from build123d import *

# Parameters (mm, degrees)
BOSS_EXTRUDE5_DEPTH = 4
SKETCH8_W           = 31.9
SKETCH8_H           = 15.8
BOSS_EXTRUDE8_DEPTH = 4.7


with BuildPart() as part:
    # Sketch1 → Boss-Extrude5 (new body)
    with BuildSketch(Plane(origin=(0, 0, 0), x_dir=(1, 0, 0), z_dir=(0, 1, 0))):
        Polygon((-17.521212205, 5.796054243), (-17.521212205, -6.003945757), (-17.521212205, -8.003945757), (14.378787795, -8.003945757), (14.378787795, -6.003945757), (14.378787795, 5.796054243), (14.378787795, 7.796054243), (-17.521212205, 7.796054243), align=None)
        with BuildLine():
            Line((-0.998289948, -2.601375998), (-1.554401677, -2.601375998))
            ThreePointArc((-1.554401677, -2.601375998), (-12.793150429, -0.101375998), (-1.554401677, 2.398624002))
            Line((-1.554401677, 2.398624002), (-0.998289948, 2.398624002))
            ThreePointArc((-0.998289948, 2.398624002), (1.501710052, -0.101375998), (-0.998289948, -2.601375998))
        make_face(mode=Mode.SUBTRACT)
    extrude(amount=BOSS_EXTRUDE5_DEPTH)

    # Sketch8 → Boss-Extrude8 (add)
    with BuildSketch(Plane(origin=(0, 4, 0), x_dir=(1, 0, 0), z_dir=(0, 1, 0))):
        with Locations((-1.571212205, -0.103945757)):
            Rectangle(SKETCH8_W, SKETCH8_H)
        Polygon((-6.895720189, 5.796054243), (-12.793150429, 5.796054243), (-12.793150429, -0.101375998), (-12.793150429, -5.998806238), (-6.895720189, -5.998806238), (9.704279811, -5.998806238), (9.704279811, 5.796054243), align=None, mode=Mode.SUBTRACT)
    extrude(amount=BOSS_EXTRUDE8_DEPTH)


solid = part.part
Design review of the part built by this model. Coordinates are the model's own, in mm. A direction names the side the tool comes from. Round coordinates to 2 decimals unless told otherwise and drop trailing zeros. Order: outer loops, then holes, each group sorted by start corner. A loop starts at its lowest first (then second) coordinate and runs counter-clockwise, first axis right, second up. Notation, with made-up numbers: M -12.5,18 L 0.5,18 A22 cw 0.5,47 Z; hole C 57.25,55.25 d4. An arc over 180 degrees is marked long. Answer as CSV lines item,"result". Start each with the question number.
1) The part is to be moulded in two halves that separate along Z. For faces 1 (the face through (9.704, 6, 0)), 2 (the face through (14.379, 4, 0)), 3 (the face through (-2, 4, 8.004)), 4 (the face through (-12.793, 6, 0)), say which applies: +Z half, -Z half, draft (parallel to the pull), parting line (faces both ways), or undercut.
2) For pin 1 Ø1.8 at (x, z) = (-10, 3) entering from +Y; pin 2 Ø6 at (x, z) = (3.5, 1) entering from +Y, all flat-tipped, find the tip position at first contact; note any pin that passes through.
3) Add section D-D (x = 8). Give the boundary of the cut face in (y, z), then the cut area to 3 significant figures.
4) Tool access review of faces 5 (the face through (1.5, 2, 0)), 6 (the face through (-2, 4, -7.796)), 7 (the face through (-2, 6, -5.796)): name each direction out of +Z, -Z, +X, -X, +Y, -Y from which nothing blocks a thin tool from reaching the whole face with its end or side.
5) Wall thickness on line 1 along Z through (x, y) = (3, 8.5); line 2 along X through (y, z) = (6.75, 3.75); line 3 along Y through (x, z) = (4, -5.25): over which ranges is each line inside the solid? List them lowest first. Write a range as [from, to].
6) Add section B-B (x = -0.5). Give the boundary of the cut face in (y, z).
7) Add section A-A (y = 6.5). Give the boundary of the cut face in (x, z), then the cut area to 3 significant figures.
Resolved:
1,face 1,"undercut"
1,face 2,"draft"
1,face 3,"+Z half"
1,face 4,"undercut"
2,pin 1,"through"
2,pin 2,"y = 4"
3,outline,"M 0,-7.8 L 8.7,-7.8 L 8.7,-5.8 L 4,-5.8 L 4,6 L 8.7,6 L 8.7,8 L 0,8 Z"
3,area,"82.0 mm^2"
4,face 5,"+Y, -Y"
4,face 6,"-Z, +X, -X, +Y, -Y"
4,face 7,"+Y"
5,line 1,"[-7.8, -5.8], [6, 8]"
5,line 2,"[-17.52, -12.79], [9.7, 14.38]"
5,line 3,"[0, 4]"
6,outline,"M 0,-7.8 L 8.7,-7.8 L 8.7,-5.8 L 4,-5.8 L 4,-2.35 L 0,-2.35 Z; M 0,2.55 L 4,2.55 L 4,6 L 8.7,6 L 8.7,8 L 0,8 Z"
7,outline,"M -17.52,-7.8 L 14.38,-7.8 L 14.38,8 L -17.52,8 Z; hole M -12.79,-5.8 L 9.7,-5.8 L 9.7,6 L -12.79,6 Z"
7,area,"239 mm^2"
